For this review, use the dimensioned drawing (mm, ordinates from the lowest corner) and the shaded views. A direction names the side the tool comes from. Round coordinates to 2 decimals unless told otherwise and drop trailing zeros. Write each loop counter-clockwise with the first axis right and the second up, starting at its lowest first coordinate (ties: lowest second). Pieces come first, ordered by that corner, then holes. Notation, with made-up numbers: (-1.75, 26.25) - (8.25, 26.25) arc R24 cw to (8.25, 59.25) - close; hole circle Ø2 at (-10, -27.75). An arc over 180 degrees is marked (long way). Return JSON: item names as keys, results as strings.
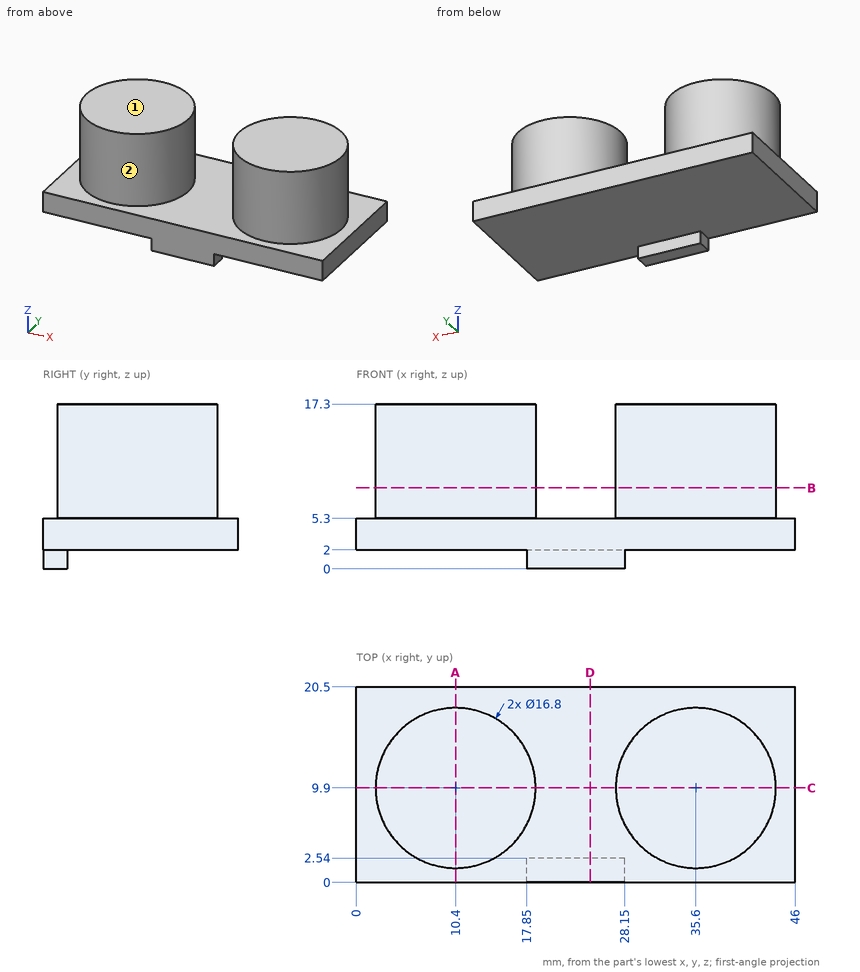
(1) Wall thickness on line 1 (Z direction, x = 40, y = 18); line 2 (Z direction, x = 10.5, y = 17.25); line 3 (X direction, y = 15.5, z = 16): over which ranges is each line inside the solid? List them lowest first.
Filled in:
{"line 1": "z = 2 to 5.3", "line 2": "z = 2 to 17.3", "line 3": "x = 4.14 to 16.66, 29.34 to 41.86"}
(2) Add section A-A (x = 10.4). Write out the cut boundary in (y, z).
Filled in:
{"outline": "(0, 2) - (20.5, 2) - (20.5, 5.3) - (18.3, 5.3) - (18.3, 17.3) - (1.5, 17.3) - (1.5, 5.3) - (0, 5.3) - close"}
(3) Clearance check with flat-ended pins moving along their axes: pin 1 Ø5 at (x, y) = (19, 5.5) entering from +Z; pin 2 Ø0.6 at (y, z) = (1, 0.5) entering from -X; pin 3 Ø0.6 at (x, z) = (24.5, 1) entering from +Y; pin 4 Ø3 at (y, z) = (16, 12.5) entering from -X. State where each tip first meets the part, or that it passes through.
Filled in:
{"pin 1": "stops at z = 17.3", "pin 2": "stops at x = 17.85", "pin 3": "stops at y = 2.54", "pin 4": "stops at x = 3.37"}
(4) Add section D-D (x = 24.5). Write out the cut boundary in (y, z).
Filled in:
{"outline": "(0, 0) - (2.54, 0) - (2.54, 2) - (20.5, 2) - (20.5, 5.3) - (0, 5.3) - close"}
(5) Add section B-B (z = 8.5). Write out the cut boundary in (x, y), plus the area to 3 significant figures.
Filled in:
{"outline": "circle Ø16.8 at (10.4, 9.9); circle Ø16.8 at (35.6, 9.9)", "area": "443 mm2"}
(6) For the marked faces 1 and 2, list the 3-axis set-ups (+Z, -Z, +X, -X, +Y, -Y) from which the entire face can be reached by the end or side of a thin tool; tool diameter is ignored.
Filled in:
{"face 1": "+Z, +X, -X, +Y, -Y", "face 2": "+Z"}
(7) Add section C-C (y = 9.9). Write out the cut boundary in (x, z).
Filled in:
{"outline": "(0, 2) - (46, 2) - (46, 5.3) - (44, 5.3) - (44, 17.3) - (27.2, 17.3) - (27.2, 5.3) - (18.8, 5.3) - (18.8, 17.3) - (2, 17.3) - (2, 5.3) - (0, 5.3) - close"}
